Could you check a few things on this model? Use its own coordinates, in mm. A direction names the side the tool comes from. Round coordinates to 2 decimals unless told otherwise and drop trailing zeros. Write each loop counter-clockwise with the first axis right and the second up, starting at its lowest first coordinate (ties: lowest second). Pieces come first, ordered by that corner, then holes. Notation, with made-up numbers: (4, 89) -> (47, 89) arc R26 ccw to (47, 120) -> close; hole circle Ø6 at (14.5, 44.25). An arc over 180 degrees is marked (long way). Return JSON: item names as keys, results as strings.
from build123d import *

# Parameters (mm, degrees)
BOSS_EXTRUDE1_DEPTH = 2
SKETCH4_R           = 1.5
CUT_EXTRUDE1_DEPTH  = 8


with BuildPart() as part:
    # Sketch2 → Revolve1 (revolve)
    with BuildSketch(Plane(origin=(0, 0, 0), x_dir=(0, 0, -1), z_dir=(1, 0, 0))):
        Polygon((-5, 0), (-5, 3), (-1.5, 3), (-1.5, 4), (-5, 4), (-5, 5), (-1, 5), (-1, 4), (1, 4), (1, 5), (5, 5), (5, 4), (1.5, 4), (1.5, 0), (0, 0), align=None)
    revolve(axis=Axis((0, 0, 7.451058405), (0, 0, -1)))

    # Sketch3 → Boss-Extrude1 (add)
    with BuildSketch(Plane(origin=(0, 0, -1.5), x_dir=(-1, 0, 0), z_dir=(0, 0, -1))):
        with BuildLine():
            ThreePointArc((1.936491673, 0.5), (1.414213562, 1.414213562), (0.5, 1.936491673))
            Line((0.5, 1.936491673), (0.5, 3.968626967))
            ThreePointArc((0.5, 3.968626967), (0, 4), (-0.5, 3.968626967))
            Line((-0.5, 3.968626967), (-0.5, 1.936491673))
            ThreePointArc((-0.5, 1.936491673), (-1.414213562, 1.414213562), (-1.936491673, 0.5))
            Line((-1.936491673, 0.5), (-3.968626967, 0.5))
            ThreePointArc((-3.968626967, 0.5), (-4, 0), (-3.968626967, -0.5))
            Line((-3.968626967, -0.5), (-1.936491673, -0.5))
            ThreePointArc((-1.936491673, -0.5), (-1.414213562, -1.414213562), (-0.5, -1.936491673))
            Line((-0.5, -1.936491673), (-0.5, -3.968626967))
            ThreePointArc((-0.5, -3.968626967), (0, -4), (0.5, -3.968626967))
            Line((0.5, -3.968626967), (0.5, -1.936491673))
            ThreePointArc((0.5, -1.936491673), (1.414213562, -1.414213562), (1.936491673, -0.5))
            Line((1.936491673, -0.5), (3.968626967, -0.5))
            ThreePointArc((3.968626967, -0.5), (3.992149037, -0.25049165), (4, 0))
            ThreePointArc((4, 0), (3.992149037, 0.25049165), (3.968626967, 0.5))
            Line((3.968626967, 0.5), (1.936491673, 0.5))
        make_face()
    extrude(amount=BOSS_EXTRUDE1_DEPTH)

    # Sketch4 → Cut-Extrude1 (cut)
    with BuildSketch(Plane.XY.offset(5)):
        Circle(SKETCH4_R)
    extrude(amount=-CUT_EXTRUDE1_DEPTH, mode=Mode.SUBTRACT)


solid = part.part
1) Will these pins go through, and if not, where does the flat tip stop? pin 1 Ø1 at (x, y) = (-2.5, -2) entering from -Z; pin 2 Ø4 at (x, y) = (0, 1) entering from -Z; pin 3 Ø1 at (y, z) = (-3, -2) entering from +X.
Return value:
{"pin 1": "z = -1.5", "pin 2": "z = -3.5", "pin 3": "x = 4.33"}
2) I want a section at D-D, the plane z = -0.75. Please give me the cut outline in (x, y), and give its area (3 significant figures).
Return value:
{"outline": "circle Ø8 at (0, 0); hole circle Ø3 at (0, 0)", "area": "43.2 mm²"}
3) If I drill on probe 1 along Z at (x, y) = (-3.75, -2.25); probe 2 along Y at (x, z) = (-2.25, -2.25); probe 3 along X at (y, z) = (1.75, 2.5), over which ranges is the centre line in solid material (lowest first)? Write a range as [from, to].
Return value:
{"probe 1": "[-5, -1], [1, 5]", "probe 2": "[-4.47, -3.31], [-0.5, 0.5], [3.31, 4.47]", "probe 3": "[-4.68, -3.6], [-2.44, 2.44], [3.6, 4.68]"}
4) Thinking about a two-plate mould opening in Y: for faces 4 (the face through (2, -2, -1.5)), 5 (the face through (-4.88, -1.08, 2.97)), which applies, pulls with the +Y half, pulls with the -Y half, needs draft (parallel to the pull), parting line crosses it, or undercut?
Return value:
{"face 4": "undercut", "face 5": "parting line crosses it"}
5) For faces 1 (the face through (3, 0.5, -2)), 2 (the face through (-3.905, -0.867, -0.014)), 3 (the face through (-3.905, -0.867, 3.274)), which set-ups out of +Z, -Z, +X, -X, +Y, -Y let a thin tool reach every point of the face, with its end or its side?
Return value:
{"face 1": "-Z", "face 2": "none", "face 3": "+Z"}
6) I want a section at A-A, the plane z = 3.5. Please give me the cut outline in (x, y).
Return value:
{"outline": "circle Ø10 at (0, 0); circle Ø6 at (0, 0); hole circle Ø8 at (0, 0); hole circle Ø3 at (0, 0)"}
7) I want a section at B-B, the plane y = 0. Please give me the cut outline in (x, z).
Return value:
{"outline": "(-5, -5) -> (-4, -5) -> (-4, -3.5) -> (4, -3.5) -> (4, -5) -> (5, -5) -> (5, -1) -> (4, -1) -> (4, 1) -> (5, 1) -> (5, 5) -> (4, 5) -> (4, 1.5) -> (3, 1.5) -> (3, 5) -> (1.5, 5) -> (1.5, -3) -> (-1.5, -3) -> (-1.5, 5) -> (-3, 5) -> (-3, 1.5) -> (-4, 1.5) -> (-4, 5) -> (-5, 5) -> (-5, 1) -> (-4, 1) -> (-4, -1) -> (-5, -1) -> close"}
